```python
from build123d import *

# Parameters (mm, degrees)
ESQUISSE1_W      = 80
ESQUISSE1_H      = 80
EXTRUSION1_DEPTH = 20
CONG_1_R         = 5
COQUE1_T         = -2


with BuildPart() as part:
    # Esquisse1 → Extrusion1 (new body)
    with BuildSketch(Plane(origin=(0, 0, 0), x_dir=(1, 0, 0), z_dir=(0, 1, 0))):
        with Locations((40, 40)):
            Rectangle(ESQUISSE1_W, ESQUISSE1_H)
    extrude(amount=EXTRUSION1_DEPTH)

    # Congé1
    cong_1_edges = [part.edges().sort_by_distance(p)[0] for p in [
        (0, 10, -80),
        (80, 10, -80),
        (80, 10, 0),
        (0, 10, 0),
    ]]
    fillet(cong_1_edges, radius=CONG_1_R)

    # Coque1
    coque1_openings = [part.faces().sort_by_distance(p)[0] for p in [
        (40, 0, -40),
    ]]
    offset(amount=COQUE1_T, openings=coque1_openings, kind=Kind.INTERSECTION)


solid = part.part
```
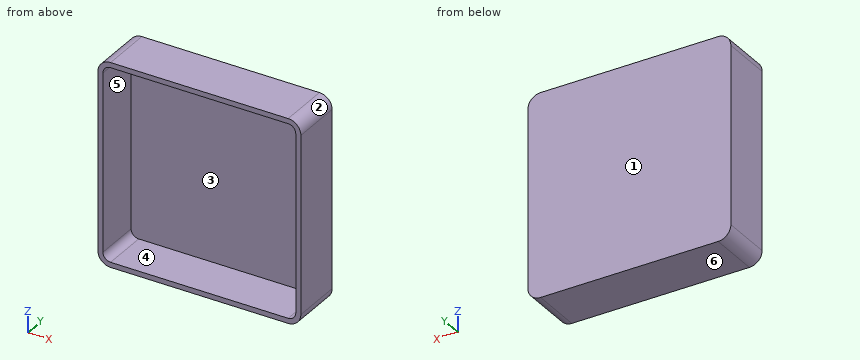
Geometry: final body of the model. Coordinates: model frame, mm. Face numbers are marked on the shaded views. A direction names the side the tool comes from. Round coordinates to 2 decimals unless told otherwise and drop trailing zeros. Loops run counter-clockwise (first coordinate to the right, second up) from the corner with the lowest first, then second, coordinate; pieces in that order, holes last. Notation, with made-up numbers: (48.5, 15.25) -> (64.5, 15.25) arc R24 cw to (64.5, 33.25) -> close; hole circle Ø7 at (84.5, -26). An arc over 180 degrees is marked (long way). Use one line per item in the form item = value. Start each with the question number.
1) First-contact query: P1, Ø6, axis at x = 19, z = -8.5, coming from the -Y side. Flat tip, straight axial feed; report the tip coordinate or a pass-through.
2) Draft query along X for the marked faces 1, 2, 3 and 4. Return one class per face: released by +X, released by -X, zero draft, split by the parting line, or undercut.
3) Section A-A on z = -49.5. Output: boundary loops of the cut face in (x, y), then the cut area to 3 significant figures.
4) Access query for the marked faces 5 and 6. Directions: +Z, -Z, +X, -X, +Y, -Y. A direction counts if a zero-diameter tool reaches every point of the face in a straight line with its end or side. Return the directions, or none.
5) Section C-C on x = 10. Output: boundary loops of the cut face in (y, z), then the cut area to 3 significant figures.
6) Section B-B on y = 3.5. Output: boundary loops of the cut face in (x, z).
7) Line query: L1, parallel to X at y = 16.5, z = -26.5; L2, parallel to Z at x = 15.5, y = 3.5; L3, parallel to Y at x = 8.5, z = -22.5. Output: solid intervals per line, ascending.
Response:
q1.P1 = 18
q2.face_1 = zero draft
q2.face_2 = released by +X
q2.face_3 = undercut
q2.face_4 = undercut
q3.outline = (0, 0) -> (2, 0) -> (2, 18) -> (78, 18) -> (78, 0) -> (80, 0) -> (80, 20) -> (0, 20) -> close
q3.area = 232 mm^2
q4.face_5 = -Y
q4.face_6 = -Z, +X, -X, +Y, -Y
q5.outline = (0, -80) -> (20, -80) -> (20, 0) -> (0, 0) -> (0, -2) -> (18, -2) -> (18, -78) -> (0, -78) -> close
q5.area = 232 mm^2
q6.outline = (0, -75) arc R5 ccw to (5, -80) -> (75, -80) arc R5 ccw to (80, -75) -> (80, -5) arc R5 ccw to (75, 0) -> (5, 0) arc R5 ccw to (0, -5) -> close; hole (2, -75) arc R3 ccw to (5, -78) -> (75, -78) arc R3 ccw to (78, -75) -> (78, -5) arc R3 ccw to (75, -2) -> (5, -2) arc R3 ccw to (2, -5) -> close
q7.L1 = 0 to 2, 78 to 80
q7.L2 = -80 to -78, -2 to 0
q7.L3 = 18 to 20
